```python
from build123d import *

# Parameters (mm, degrees)
ESQUISSE1_W             = 130
ESQUISSE1_H             = 100
BOSS_EXTRU_1_DEPTH      = 5
ESQUISSE2_R             = 1.75
ENL_V_MAT_EXTRU_1_DEPTH = 10
ESQUISSE4_W             = 19.900527691
ESQUISSE4_H             = 30
ENL_V_MAT_EXTRU_2_DEPTH = 10
CONG_1_R                = 5


with BuildPart() as part:
    # Esquisse1 → Boss.-Extru.1 (new body)
    with BuildSketch(Plane.XY):
        with Locations((-11.008064516, 2.681451613)):
            Rectangle(ESQUISSE1_W, ESQUISSE1_H)
    extrude(amount=BOSS_EXTRU_1_DEPTH)

    # Esquisse2 → Enlèv. mat.-Extru.1 (cut)
    with BuildSketch(Plane.XY.offset(5)):
        with Locations((9.851585529, -18.178198432)):
            Circle(ESQUISSE2_R)
        with Locations((-31.867714561, -18.178198432)):
            Circle(ESQUISSE2_R)
        with Locations((-31.867714561, 23.541101658)):
            Circle(ESQUISSE2_R)
        with Locations((9.851585529, 23.541101658)):
            Circle(ESQUISSE2_R)
    extrude(amount=-ENL_V_MAT_EXTRU_1_DEPTH, mode=Mode.SUBTRACT)

    # Esquisse4 → Enlèv. mat.-Extru.2 (cut)
    with BuildSketch(Plane.XY.offset(5)):
        with Locations((-66.057800671, 2.681451613)):
            Rectangle(ESQUISSE4_W, ESQUISSE4_H)
    extrude(amount=-ENL_V_MAT_EXTRU_2_DEPTH, mode=Mode.SUBTRACT)

    # Congé1
    cong_1_edges = [part.edges().sort_by_distance(p)[0] for p in [
        (-56.107536825, 17.681451613, 2.5),
        (-56.107536825, -12.318548387, 2.5),
        (-76.008064516, 52.681451613, 2.5),
        (53.991935484, 52.681451613, 2.5),
        (53.991935484, -47.318548387, 2.5),
        (-76.008064516, -47.318548387, 2.5),
    ]]
    fillet(cong_1_edges, radius=CONG_1_R)


solid = part.part
```
Geometry check sheet. Reference: the model listing, model coordinates, mm. A direction names the side the tool comes from. Give positions to 0.01 mm unless a question says otherwise; leave off trailing zeros. Order: outer loops, then holes, each group sorted by start corner. A loop starts at its lowest first (then second) coordinate and runs counter-clockwise, first axis right, second up. Notation, with made-up numbers: (-7.5, 73) -> (26.5, 73) arc R13 cw to (26.5, 84) -> close; hole circle Ø2 at (50, 82). An arc over 180 degrees is marked (long way). Write each question's results on one line, items separated by ' | '. Start each with the question number.
(1) Sectioned sample at B-B (y = 2.5). Enter the section's corners in (x, z).
(2) Mould release check, pull along Y, two halves, no side actions. Record for faces 1 (the face through (-12, 3, 0)), 2 (the face through (52.488, 51.256, 2.535)), 3 (the face through (-57.533, 16.178, 2.465)): pulls with the +Y half, pulls with the -Y half, needs draft (parallel to the pull), parting line crosses it, or undercut.
(3) Scan lines: line 1 (Y direction, x = -61, z = 4.65); line 2 (Y direction, x = 10.5, z = 1); line 3 (X direction, y = -3.5, z = 4.7). Record each from-to range of solid material in increasing order.
(4) Access from +Z, -Z, +X, -X, +Y, -Y to the whole of each face (thin tool, end or side, straight path). Record for faces 4 (the face through (-74.58, 51.18, 2.54)), 5 (the face through (-56.108, 3, 3)).
(5) Gauge pin test, flat ends, axial feed: P1, Ø5.5, axis at x = 9.85, y = -18.18, coming from the +Z side; P2, Ø3, axis at x = -31.87, y = -18.18, coming from the +Z side; P3, Ø1.5, axis at y = 3.5, z = 2.5, coming from the -X side. Record the tip position at first contact, or that the pin passes through.
(6) Sectioned sample at A-A (z = 1.85). Enter the section's corners in (x, y).
Answer below:
1) outline: (-56.11, 0) -> (53.99, 0) -> (53.99, 5) -> (-56.11, 5) -> close
2) face 1: needs draft | face 2: pulls with the +Y half | face 3: undercut
3) line 1: -47.32 to -12.32, 17.68 to 52.68 | line 2: -47.32 to -19.8, -16.55 to 21.92, 25.17 to 52.68 | line 3: -56.11 to 53.99
4) face 4: +Z, -Z, -X, +Y | face 5: +Z, -Z, -X
5) P1: z = 5 | P2: through | P3: x = -56.11
6) outline: (-76.01, -42.32) arc R5 ccw to (-71.01, -47.32) -> (48.99, -47.32) arc R5 ccw to (53.99, -42.32) -> (53.99, 47.68) arc R5 ccw to (48.99, 52.68) -> (-71.01, 52.68) arc R5 ccw to (-76.01, 47.68) -> (-76.01, 17.68) -> (-61.11, 17.68) arc R5 cw to (-56.11, 12.68) -> (-56.11, -7.32) arc R5 cw to (-61.11, -12.32) -> (-76.01, -12.32) -> close; hole circle Ø3.5 at (-31.87, -18.18); hole circle Ø3.5 at (-31.87, 23.54); hole circle Ø3.5 at (9.85, -18.18); hole circle Ø3.5 at (9.85, 23.54)
